The model under review builds one solid part; all positions refer to its coordinate system, in mm. Face numbers are marked on the shaded views. A direction names the side the tool comes from. Give positions to 0.01 mm unless a question says otherwise; leave off trailing zeros. Order: outer loops, then holes, each group sorted by start corner. A loop starts at its lowest first (then second) coordinate and runs counter-clockwise, first axis right, second up.
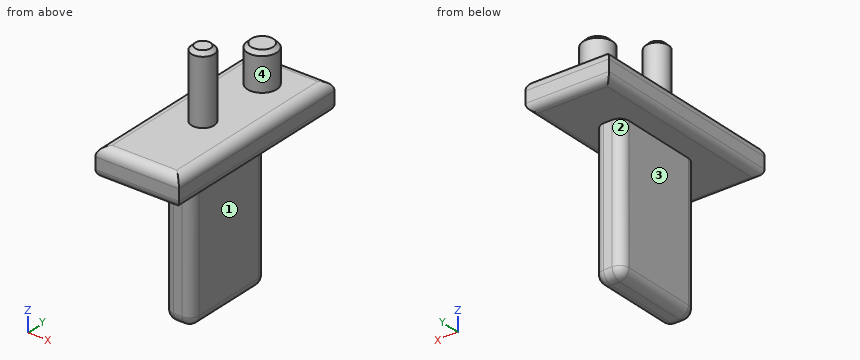
```python
from build123d import *

# Parameters (mm, degrees)
F0_W     = 11.176
F0_H     = 26.67
F1_DEPTH = 3.81
F2_R     = 1.9685
F3_DEPTH = 4.953
F2_R_2   = 1.524
F4_DEPTH = 9.144
F5_SIZE  = 0.508
F6_R     = 1.27
F7_R     = 1.016
F8_W     = 3.683
F8_H     = 12.7
F9_DEPTH = 19.05
F10_R    = 1.27


with BuildPart() as f1:
    # F0 (on Top) → F1 (new body)
    with BuildSketch(Plane.XY):
        Rectangle(F0_W, F0_H)
    extrude(amount=F1_DEPTH)

    # F2 (on face) → F3 (join)
    with BuildSketch(Plane.XY.offset(3.81)):
        with Locations((0, 8.0772)):
            Circle(F2_R)
    extrude(amount=F3_DEPTH)

    # F2 (on face) → F4 (join)
    with BuildSketch(Plane.XY.offset(3.81)):
        with Locations((0, -2.0828)):
            Circle(F2_R_2)
    extrude(amount=F4_DEPTH)

    # F5
    f5_edges = [f1.edges().sort_by_distance(p)[0] for p in [
        (-1.9685, 8.0772, 8.763),
        (-1.524, -2.0828, 12.954),
    ]]
    chamfer(f5_edges, length=F5_SIZE)

    # F6
    f6_edges = [f1.edges().sort_by_distance(p)[0] for p in [
        (0, 13.335, 3.81),
        (5.588, 0, 3.81),
        (0, -13.335, 3.81),
        (-5.588, 0, 3.81),
    ]]
    fillet(f6_edges, radius=F6_R)

    # F7
    f7_edges = [f1.edges().sort_by_distance(p)[0] for p in [
        (0, 13.335, 0),
        (5.588, 0, 0),
        (0, -13.335, 0),
        (-5.588, 0, 0),
    ]]
    fillet(f7_edges, radius=F7_R)

    # F8 (on face) → F9 (join)
    with BuildSketch(Plane(origin=(0, 0, 0), x_dir=(1, 0, 0), z_dir=(0, 0, -1))):
        Rectangle(F8_W, F8_H)
    extrude(amount=F9_DEPTH)

    # F10
    f10_edges = [f1.edges().sort_by_distance(p)[0] for p in [
        (0, -6.35, -19.05),
        (-1.8415, 0, -19.05),
        (1.8415, 0, -19.05),
        (0, 6.35, -19.05),
        (-1.8415, -6.35, -9.525),
        (1.8415, -6.35, -9.525),
        (1.8415, 6.35, -9.525),
        (-1.8415, 6.35, -9.525),
    ]]
    fillet(f10_edges, radius=F10_R)


solid = f1.part
```
Item 1: For the marked faces 1, 2, 3 and 4, list the 3-axis set-ups (+Z, -Z, +X, -X, +Y, -Y) from which the entire face can be reached by the end or side of a thin tool; tool diameter is ignored.
Values found:
face 1: -Z, +X, +Y, -Y
face 2: -Z, -X, +Y
face 3: -Z, -X, +Y, -Y
face 4: +Z
Item 2: Clearance check with flat-ended pins moving along their axes: pin 1 Ø5 at (x, y) = (-3, 7) entering from +Z; pin 2 Ø5 at (y, z) = (5, -12) entering from -X; pin 3 Ø10 at (y, z) = (8, -10) entering from +X; pin 4 Ø1 at (y, z) = (8, -4.5) entering from -X. State where each tip first meets the part, or that it passes through.
Values found:
pin 1: stops at z = 8.76
pin 2: stops at x = -1.84
pin 3: stops at x = 1.84
pin 4: passes through
Item 3: For line 1 (Z direction, x = -3.5, y = 1.5); line 2 (X direction, y = -2.75, z = -12.5); line 3 (Y direction, x = 1, z = 5), list the stretches that pass through material, from the lowest coordinate up.
Values found:
line 1: z = 0 to 3.81
line 2: x = -1.84 to 1.84
line 3: y = -3.23 to -0.93, 6.38 to 9.77
Item 4: Take a section at A-A (y = -4.25). Give the boundary of the cut face in (x, z), and give its area (3 significant figures).
Values found:
outline: (-5.59, 1.02) arc R1.02 ccw to (-4.57, 0) - (-1.84, 0) - (-1.84, -17.78) arc R1.27 ccw to (-0.57, -19.05) - (0.57, -19.05) arc R1.27 ccw to (1.84, -17.78) - (1.84, 0) - (4.57, 0) arc R1.02 ccw to (5.59, 1.02) - (5.59, 2.54) arc R1.27 ccw to (4.32, 3.81) - (-4.32, 3.81) arc R1.27 ccw to (-5.59, 2.54) - close
area: 111 mm2
Item 5: Take a section at C-C (x = -3.25). Give the boundary of the cut face in (y, z) (3 decimals), and give its area (3 significant figures).
Values found:
outline: (-13.335, 1.016) arc R1.016 ccw to (-12.319, 0) - (12.319, 0) arc R1.016 ccw to (13.335, 1.016) - (13.335, 2.54) arc R1.27 ccw to (12.065, 3.81) - (-12.065, 3.81) arc R1.27 ccw to (-13.335, 2.54) - close
area: 100 mm2
Item 6: Take a section at B-B (z = -2). Give the boundary of the cut face in (x, y).
Values found:
outline: (-1.84, -5.08) arc R1.27 ccw to (-0.57, -6.35) - (0.57, -6.35) arc R1.27 ccw to (1.84, -5.08) - (1.84, 5.08) arc R1.27 ccw to (0.57, 6.35) - (-0.57, 6.35) arc R1.27 ccw to (-1.84, 5.08) - close
Item 7: Take a section at D-D (x = 0). Give the boundary of the cut face in (y, z) (3 decimals), and give its area (3 significant figures).
Values found:
outline: (-13.335, 1.016) arc R1.016 ccw to (-12.319, 0) - (-6.35, 0) - (-6.35, -17.78) arc R1.27 ccw to (-5.08, -19.05) - (5.08, -19.05) arc R1.27 ccw to (6.35, -17.78) - (6.35, 0) - (12.319, 0) arc R1.016 ccw to (13.335, 1.016) - (13.335, 2.54) arc R1.27 ccw to (12.065, 3.81) - (10.046, 3.81) - (10.046, 8.255) - (9.538, 8.763) - (6.617, 8.763) - (6.109, 8.255) - (6.109, 3.81) - (-0.559, 3.81) - (-0.559, 12.446) - (-1.067, 12.954) - (-3.099, 12.954) - (-3.607, 12.446) - (-3.607, 3.81) - (-12.065, 3.81) arc R1.27 ccw to (-13.335, 2.54) - close
area: 389 mm2
